Here's how the part is built. I have some questions about the finished solid (model axes, mm). Face numbers are marked on the shaded views. A direction names the side the tool comes from. Round coordinates to 2 decimals unless told otherwise and drop trailing zeros. Order: outer loops, then holes, each group sorted by start corner. A loop starts at its lowest first (then second) coordinate and runs counter-clockwise, first axis right, second up. Notation, with made-up numbers: (-5.5, 37.25) -> (44.5, 37.25) arc R19 ccw to (44.5, 57.25) -> close; hole circle Ø5 at (-20, -2). An arc over 180 degrees is marked (long way). Answer in a Markdown table with one row per item.
```python
from build123d import *

# Parameters (mm, degrees)
SZKIC1_R                    = 1.55
DODANIE_WYCI_GNI_CIE1_DEPTH = 6
DODANIE_WYCI_GNI_CIE2_DEPTH = 6
WYTNIJ_WYCI_GNI_CIE3_START  = -10
SZKIC2_R                    = 0.665
SZKIC2_R_2                  = 1.55
WYTNIJ_WYCI_GNI_CIE3_DEPTH  = 10
SZYK_LINIOWY1_OUTLINE_R     = 0.665
SZYK_LINIOWY1_DEPTH         = 6
SZKIC6_R                    = 1.55
WYTNIJ_WYCI_GNI_CIE6_DEPTH  = 6


# Read off the part's stored shape, not the designer's step: Szyk liniowy1
with BuildPart() as part:
    # Szkic1 → Dodanie-wyciągnięcie1 (new body)
    with BuildSketch(Plane.XY):
        with BuildLine():
            Line((-166.275426397, 1549.053482816), (-188.475426397, 1549.053482816))
            ThreePointArc((-188.475426397, 1549.053482816), (-192.475426397, 1553.053482816), (-188.475426397, 1557.053482816))
            Line((-188.475426397, 1557.053482816), (-166.275426397, 1557.053482816))
            ThreePointArc((-166.275426397, 1557.053482816), (-162.275426397, 1553.053482816), (-166.275426397, 1549.053482816))
        make_face()
        with Locations((-166.275426397, 1553.053482816)):
            Circle(SZKIC1_R, mode=Mode.SUBTRACT)
    extrude(amount=DODANIE_WYCI_GNI_CIE1_DEPTH)

    # Szkic5 → Dodanie-wyciągnięcie2 (add)
    with BuildSketch(Plane.XY.offset(6)):
        with BuildLine():
            Line((-195.475426397, 1563.495915282), (-195.475426397, 1563.574683951))
            ThreePointArc((-195.475426397, 1563.574683951), (-194.81837577, 1565.056738938), (-193.278939414, 1565.565008766))
            Line((-193.278939414, 1565.565008766), (-191.112699272, 1565.351155235))
            Line((-191.112699272, 1565.351155235), (-184.565954248, 1564.704853604))
            ThreePointArc((-184.565954248, 1564.704853604), (-182.02952048, 1563.221328031), (-181.029706775, 1560.458228876))
            Line((-181.029706775, 1560.458228876), (-181.029706775, 1560.053482816))
            ThreePointArc((-181.029706775, 1560.053482816), (-180.151027119, 1557.932162472), (-178.029706775, 1557.053482816))
            Line((-178.029706775, 1557.053482816), (-178.029706775, 1549.053482816))
            ThreePointArc((-178.029706775, 1549.053482816), (-180.151027119, 1548.174803159), (-181.029706775, 1546.053482816))
            Line((-181.029706775, 1546.053482816), (-181.029706775, 1545.648736756))
            ThreePointArc((-181.029706775, 1545.648736756), (-181.939081075, 1542.810326939), (-184.565954248, 1541.402112028))
            Line((-184.565954248, 1541.402112028), (-188.141654627, 1541.049115084))
            Line((-188.141654627, 1541.049115084), (-193.278939414, 1540.541956866))
            ThreePointArc((-193.278939414, 1540.541956866), (-194.81837577, 1541.050226694), (-195.475426397, 1542.53228168))
            Line((-195.475426397, 1542.53228168), (-195.475426397, 1542.61105035))
            ThreePointArc((-195.475426397, 1542.61105035), (-195.242164639, 1544.267773032), (-194.560516381, 1545.795679033))
            ThreePointArc((-194.560516381, 1545.795679033), (-192.475426397, 1553.053482816), (-194.560516381, 1560.311286599))
            ThreePointArc((-194.560516381, 1560.311286599), (-195.242164639, 1561.839192599), (-195.475426397, 1563.495915282))
        make_face()
    extrude(amount=-DODANIE_WYCI_GNI_CIE2_DEPTH)

    # Szkic2 → Wytnij-wyciągnięcie3 (cut)
    with BuildSketch(Plane.XY.offset(6).offset(WYTNIJ_WYCI_GNI_CIE3_START)):
        with Locations((-188.475426397, 1553.053482816)):
            Circle(SZKIC2_R)
        with Locations((-166.275426397, 1553.053482816)):
            Circle(SZKIC2_R_2)
    extrude(amount=WYTNIJ_WYCI_GNI_CIE3_DEPTH, mode=Mode.SUBTRACT)

    # Szyk liniowy1 outline → Szyk liniowy1 (cut)
    with BuildSketch(Plane.XY):
        with Locations((-185.475426397, 1553.053482816)):
            Circle(SZYK_LINIOWY1_OUTLINE_R)
        with Locations((-182.475426397, 1553.053482816)):
            Circle(SZYK_LINIOWY1_OUTLINE_R)
        with Locations((-179.475426397, 1553.053482816)):
            Circle(SZYK_LINIOWY1_OUTLINE_R)
        with Locations((-176.475426397, 1553.053482816)):
            Circle(SZYK_LINIOWY1_OUTLINE_R)
    extrude(amount=SZYK_LINIOWY1_DEPTH, mode=Mode.SUBTRACT)

    # Szkic6 → Wytnij-wyciągnięcie6 (cut)
    with BuildSketch(Plane(origin=(0, 0, 0), x_dir=(-1, 0, 0), z_dir=(0, 0, -1))):
        with Locations((185.004427547, 1560.742573003)):
            Circle(SZKIC6_R)
        with Locations((191.475426395, 1561.355903175)):
            Circle(SZKIC6_R)
        with Locations(Location((191.475426395, 1545.035406583, 0), (0, 0, 180))):
            Circle(SZKIC6_R)
        with Locations(Location((185.004427547, 1545.648736756, 0), (0, 0, 180))):
            Circle(SZKIC6_R)
    extrude(amount=-WYTNIJ_WYCI_GNI_CIE6_DEPTH, mode=Mode.SUBTRACT)


solid = part.part
```
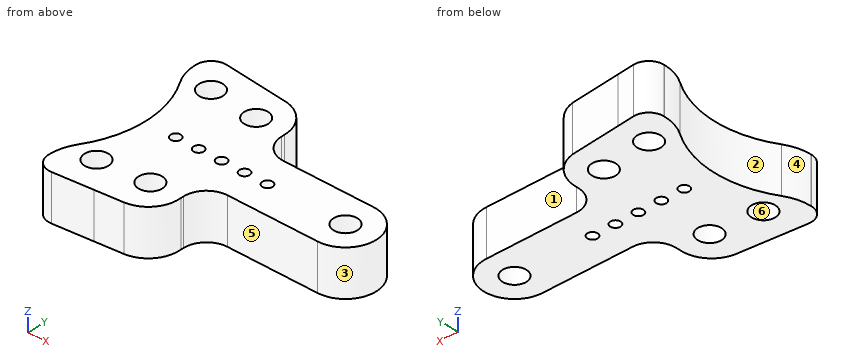
1. For pin 1 Ø4 at (x, y) = (-191.48, 1561.36) entering from -Z; pin 2 Ø1.8 at (x, z) = (-172, 4) entering from -Y; pin 3 Ø3 at (x, z) = (-171, 3) entering from +Y; pin 4 Ø3 at (y, z) = (1548.5, 2.5) entering from +X, each with a flat end and sliding along its axis, tell me the tip position at first contact or that it passes through.
Numbers:
| item | result |
|---|---|
| pin 1 | stops at z = 0 |
| pin 2 | stops at y = 1549.05 |
| pin 3 | stops at y = 1557.05 |
| pin 4 | stops at x = -163.69 |
2. Suppose I cut it at D-D on y = 1555.75. Write out the boundary of the cut face in (x, z), then the cut area to 3 significant figures.
Numbers:
| item | result |
|---|---|
| outline | (-192.74, 0) -> (-163.32, 0) -> (-163.32, 6) -> (-192.74, 6) -> close |
| area | 177 mm2 |
3. Please list where these lines run through material, in increasing order: line 1 along Y through (x, z) = (-185.5, 0.3); line 2 along X through (y, z) = (1562, 3.95); line 3 along X through (y, z) = (1560.5, 1.8).
Numbers:
| item | result |
|---|---|
| line 1 | y = 1541.31 to 1544.18, 1547.12 to 1552.39, 1553.72 to 1559.27, 1562.21 to 1564.8 |
| line 2 | x = -195.29 to -192.89, -190.07 to -185.91, -184.1 to -181.31 |
| line 3 | x = -194.67 to -192.77, -190.18 to -186.54, -183.47 to -181.03 |
4. We'd pull the mould along Y, two halves only. Please class the marked faces 1, 2 and 3: released by +Y, released by -Y, zero draft, split by the parting line, or undercut.
Numbers:
| item | result |
|---|---|
| face 1 | released by +Y |
| face 2 | undercut |
| face 3 | split by the parting line |
5. Suppose I cut it at A-A on y = 1552. Write out the boundary of the cut face in (x, z), then the cut area to 3 significant figures.
Numbers:
| item | result |
|---|---|
| outline | (-192.52, 0) -> (-167.41, 0) -> (-167.41, 6) -> (-192.52, 6) -> close; (-165.14, 0) -> (-162.42, 0) -> (-162.42, 6) -> (-165.14, 6) -> close |
| area | 167 mm2 |
6. Suppose I cut it at B-B on z = 3.95. State how many separate pieces and enclosed holes the cut face has, then the cut area to 3 significant figures.
Numbers:
| item | result |
|---|---|
| separate pieces | 1 |
| enclosed holes | 10 |
| area | 406 mm2 |
7. Suppose I cut it at C-C on x = -169.5. Write out the boundary of the cut face in (y, z), then the cut area to 3 significant figures.
Numbers:
| item | result |
|---|---|
| outline | (1549.05, 0) -> (1557.05, 0) -> (1557.05, 6) -> (1549.05, 6) -> close |
| area | 48.0 mm2 |
8. For the marked faces 4, 5 and 6, which set-ups out of +Z, -Z, +X, -X, +Y, -Y let a thin tool reach every point of the face, with its end or its side?
Numbers:
| item | result |
|---|---|
| face 4 | +Z, -Z, -X |
| face 5 | +Z, -Z, +X, -Y |
| face 6 | +Z, -Z |
